The model under review builds one solid part; all positions refer to its coordinate system, in mm. Face numbers are marked on the shaded views. Round coordinates to 2 decimals unless told otherwise and drop trailing zeros. Order: outer loops, then holes, each group sorted by start corner. A loop starts at its lowest first (then second) coordinate and runs counter-clockwise, first axis right, second up. Notation, with made-up numbers: M -23.75,27 L 21.25,27 A25 cw 21.25,56 Z; hole C 13,51.25 d7. An arc over 180 degrees is marked long. Use a Markdown table: item, result. Add a question column.
1. Insertion check: P1, Ø4, axis at x = 38.5, y = 4.5, coming from the +Z side; P2, Ø6.5, axis at x = 45, z = 0, coming from the -Y side; P3, Ø5, axis at y = 5, z = 35, coming from the +X side. Each pin has a flat end and moves straight along its axis. Give the tip position at first contact, or say it passes through.
2. Consider section D-D on z = 45. State the section outline as (x, y) points, then the cut area to 3 significant figures.
3. Consider section C-C on y = 16.25. State the section outline as (x, z) points, then the cut area to 3 significant figures.
4. The part is to be moulded in two halves that separate along Z. For the marked faces 1, 2, 3 and 4, say which applies: +Z half, -Z half, draft (parallel to the pull), parting line (faces both ways), or undercut.
5. Consider section B-B on z = 0. State the section outline as (x, y) points, then the cut area to 3 significant figures.
6. To check wall thickness, follow probe 1 along Z at (x, y) = (0, 3.9); probe 2 along Z at (x, y) = (0, 14.75). State the ranges of each line that lie inside material, in increasing order.
7. Consider section A-A on x = 0. State the section outline as (y, z) points.
from build123d import *

# Parameters (mm, degrees)
SKETCH1_R           = 55
SKETCH1_R_2         = 14.5
BOSS_EXTRUDE1_DEPTH = 20
SKETCH2_R           = 21.2
CUT_EXTRUDE1_DEPTH  = 10
SKETCH4_R           = 2
CUT_EXTRUDE2_DEPTH  = 20
SKETCH6_R           = 5
CUT_EXTRUDE3_DEPTH  = 5


with BuildPart() as part:
    # Sketch1 → Boss-Extrude1 (new body)
    with BuildSketch(Plane(origin=(0, 0, 0), x_dir=(1, 0, 0), z_dir=(0, 1, 0))):
        Circle(SKETCH1_R)
        Circle(SKETCH1_R_2, mode=Mode.SUBTRACT)
    extrude(amount=BOSS_EXTRUDE1_DEPTH)

    # Sketch2 → Cut-Extrude1 (cut)
    with BuildSketch(Plane(origin=(0, 20, 0), x_dir=(1, 0, 0), z_dir=(0, 1, 0))):
        Circle(SKETCH2_R)
    extrude(amount=-CUT_EXTRUDE1_DEPTH, mode=Mode.SUBTRACT)

    # Sketch4 → Cut-Extrude2 (cut)
    with BuildSketch(Plane(origin=(0, 20, 0), x_dir=(1, 0, 0), z_dir=(0, 1, 0))):
        with Locations((0, 45)):
            Circle(SKETCH4_R)
        with Locations((45, 0)):
            Circle(SKETCH4_R)
        with Locations((0, -45)):
            Circle(SKETCH4_R)
        with Locations((-45, 0)):
            Circle(SKETCH4_R)
    extrude(amount=-CUT_EXTRUDE2_DEPTH, mode=Mode.SUBTRACT)

    # Sketch6 → Cut-Extrude3 (cut)
    with BuildSketch(Plane.XZ):
        with Locations((0, 45)):
            Circle(SKETCH6_R)
        with Locations((45, 0)):
            Circle(SKETCH6_R)
        with Locations((0, -45)):
            Circle(SKETCH6_R)
        with Locations((-45, 0)):
            Circle(SKETCH6_R)
    extrude(amount=-CUT_EXTRUDE3_DEPTH, mode=Mode.SUBTRACT)


solid = part.part
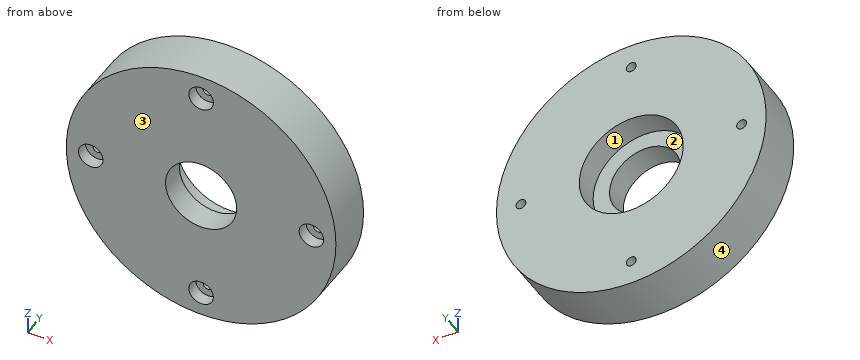
Answer block:
| question | item | result |
|---|---|---|
| 1 | P1 | z = 41.14 |
| 1 | P2 | y = 5 |
| 1 | P3 | x = 44.37 |
| 2 | outline | M -31.62,0 L -5,0 L -5,5 L -2,5 L -2,20 L -31.62,20 Z; M 2,5 L 5,5 L 5,0 L 31.62,0 L 31.62,20 L 2,20 Z |
| 2 | area | 1,150 mm^2 |
| 3 | outline | C 0,0 d110; hole C -45,0 d4; hole C 0,0 d42.4; hole C 0,-45 d4; hole C 0,45 d4; hole C 45,0 d4 |
| 3 | area | 8,040 mm^2 |
| 4 | face 1 | undercut |
| 4 | face 2 | undercut |
| 4 | face 3 | draft |
| 4 | face 4 | parting line |
| 5 | outline | M -55,0 L -50,0 L -50,5 L -47,5 L -47,20 L -55,20 Z; M -43,5 L -40,5 L -40,0 L -14.5,0 L -14.5,10 L -21.2,10 L -21.2,20 L -43,20 Z; M 14.5,0 L 40,0 L 40,5 L 43,5 L 43,20 L 21.2,20 L 21.2,10 L 14.5,10 Z; M 47,5 L 50,5 L 50,0 L 55,0 L 55,20 L 47,20 Z |
| 5 | area | 1,270 mm^2 |
| 6 | probe 1 | -55 to -50, -40 to -14.5, 14.5 to 40, 50 to 55 |
| 6 | probe 2 | -55 to -47, -43 to -21.2, 21.2 to 43, 47 to 55 |
| 7 | outline | M 0,-55 L 20,-55 L 20,-47 L 5,-47 L 5,-50 L 0,-50 Z; M 0,-40 L 5,-40 L 5,-43 L 20,-43 L 20,-21.2 L 10,-21.2 L 10,-14.5 L 0,-14.5 Z; M 0,14.5 L 10,14.5 L 10,21.2 L 20,21.2 L 20,43 L 5,43 L 5,40 L 0,40 Z; M 0,50 L 5,50 L 5,47 L 20,47 L 20,55 L 0,55 Z |
